Geometry check sheet. Reference: the model listing, model coordinates, mm. A direction names the side the tool comes from. Round coordinates to 2 decimals unless told otherwise and drop trailing zeros. Write each loop counter-clockwise with the first axis right and the second up, starting at its lowest first coordinate (ties: lowest second). Pieces come first, ordered by that corner, then holes.
Item 1: Cross-section at C-C (z = 43). Enter the section's corners in (x, y), then the cut area to 3 significant figures.
Item 2: Cross-section at B-B (y = 0). Enter the section's corners in (x, z), then the cut area to 3 significant figures.
Item 3: Scan lines: probe 1 along Z at (x, y) = (-1.25, -2.5); probe 2 along Z at (x, y) = (8.5, 0); probe 3 along Y at (x, z) = (8.5, 49.25). Record each from-to range of solid material in increasing order.
Item 4: Depth check by flat-ended pin: P1, Ø6, axis at y = -6.5, z = 42.5, coming from the +X side; P2, Ø4, axis at y = -8, z = 35, coming from the +X side; P3, Ø2, axis at x = -5, z = 48, coming from the -Y side. Enter the tip coordinate at first touch or a pass-through.
Item 5: Cross-section at A-A (x = 0). Enter the section's corners in (y, z), then the cut area to 3 significant figures.
Item 6: Cross-section at D-D (y = 10). Enter the section's corners in (x, z).
Item 7: Draft check along Y on faces 1 (the face through (-10, 0, 51)), 2 (the face through (7.3, -0.9, 51.3)), 3 (the face through (0, 0, 0)), 4 (the face through (11.923, 3.755, 28.402)). Enter one of: pulls with the +Y half, pulls with the -Y half, needs draft (parallel to the pull), parting line crosses it, or undercut.
Item 8: Access from +Z, -Z, +X, -X, +Y, -Y to the whole of each face (thin tool, end or side, straight path). Record for faces 5 (the face through (-9, 0, 44.91)), 6 (the face through (0, 0, 75.61)).
from build123d import *

# Parameters (mm, degrees)
F0_R     = 12.5
F1_DEPTH = 57.61
F2_R     = 2
F3_DEPTH = 18
F4_R     = 1.5
F5_DEPTH = 12.7


with BuildPart() as f1:
    # F0 (on Top) → F1 (new body)
    with BuildSketch(Plane.XY):
        Circle(F0_R)
    extrude(amount=F1_DEPTH)

    # F2 (on face) → F3 (join)
    with BuildSketch(Plane.XY.offset(57.61)):
        Circle(F2_R)
    extrude(amount=F3_DEPTH)

    # F4 (on face) → F5 (cut)
    with BuildSketch(Plane.XY.offset(57.61)):
        with Locations((-8.5, 0)):
            Circle(F4_R)
        with Locations((8.5, 0)):
            Circle(F4_R)
    extrude(amount=-F5_DEPTH, mode=Mode.SUBTRACT)


solid = f1.part
Resolved:
1. outline: circle Ø25 at (0, 0)
1. area: 491 mm2
2. outline: (-12.5, 0) - (12.5, 0) - (12.5, 57.61) - (10, 57.61) - (10, 44.91) - (7, 44.91) - (7, 57.61) - (2, 57.61) - (2, 75.61) - (-2, 75.61) - (-2, 57.61) - (-7, 57.61) - (-7, 44.91) - (-10, 44.91) - (-10, 57.61) - (-12.5, 57.61) - close
2. area: 1,440 mm2
3. probe 1: z = 0 to 57.61
3. probe 2: z = 0 to 44.91
3. probe 3: y = -9.17 to -1.5, 1.5 to 9.17
4. P1: stops at x = 12
4. P2: stops at x = 10.97
4. P3: stops at y = -11.84
5. outline: (-12.5, 0) - (12.5, 0) - (12.5, 57.61) - (2, 57.61) - (2, 75.61) - (-2, 75.61) - (-2, 57.61) - (-12.5, 57.61) - close
5. area: 1,510 mm2
6. outline: (-7.5, 0) - (7.5, 0) - (7.5, 57.61) - (-7.5, 57.61) - close
7. face 1: undercut
7. face 2: undercut
7. face 3: needs draft
7. face 4: parting line crosses it
8. face 5: +Z
8. face 6: +Z, +X, -X, +Y, -Y
